Can you work these out from the drawing? Everything is in mm from the part's minimum corner. A direction names the side the tool comes from. Give positions to 0.01 mm unless a question says otherwise; leave off trailing zeros. Loops run counter-clockwise (first coordinate to the right, second up) from the corner with the lowest first, then second, coordinate; pieces in that order, holes last.
Q1. For the marked faces 4, 5, 6, 7 and 8, which set-ups out of +Z, -Z, +X, -X, +Y, -Y let a thin tool reach every point of the face, with its end or its side?
Q2. Will these pins go through, and if not, where does the flat tip stop? P1, Ø23.5, axis at x = 88, z = 17, coming from the -Y side (1 decimal); P2, Ø3, axis at y = 24.5, z = 14, coming from the -X side (1 decimal); P3, Ø8, axis at x = 99.5, z = 9.5, coming from the +Y side (1 decimal).
Q3. I need wall thicknesses on line 1 (Y direction, x = 115, z = 34) (1 decimal); line 2 (Z direction, x = 47, y = 15); line 3 (Y direction, x = 21.15, z = 6.5) (1 decimal). Which ranges of each line are inside material? Lowest first, please.
Q4. We'd pull the mould along Y, two halves only. Please class the marked faces 1, 2 and 3: +Y half, -Y half, draft (parallel to the pull), parting line (faces both ways), or undercut.
Q5. If we section it at D-D (z = 36): Please give me the cut outline in (x, y) (1 decimal), plus the area to 3 significant figures.
Q6. If we section it at C-C (y = 17.5): Please give me the cut outline in (x, z) (1 decimal).
Q7. If we section it at B-B (x = 21.15): Please give me the cut outline in (y, z) (1 decimal).
Q8. If we section it at A-A (y = 25.5): Please give me the cut outline in (x, z) (1 decimal).
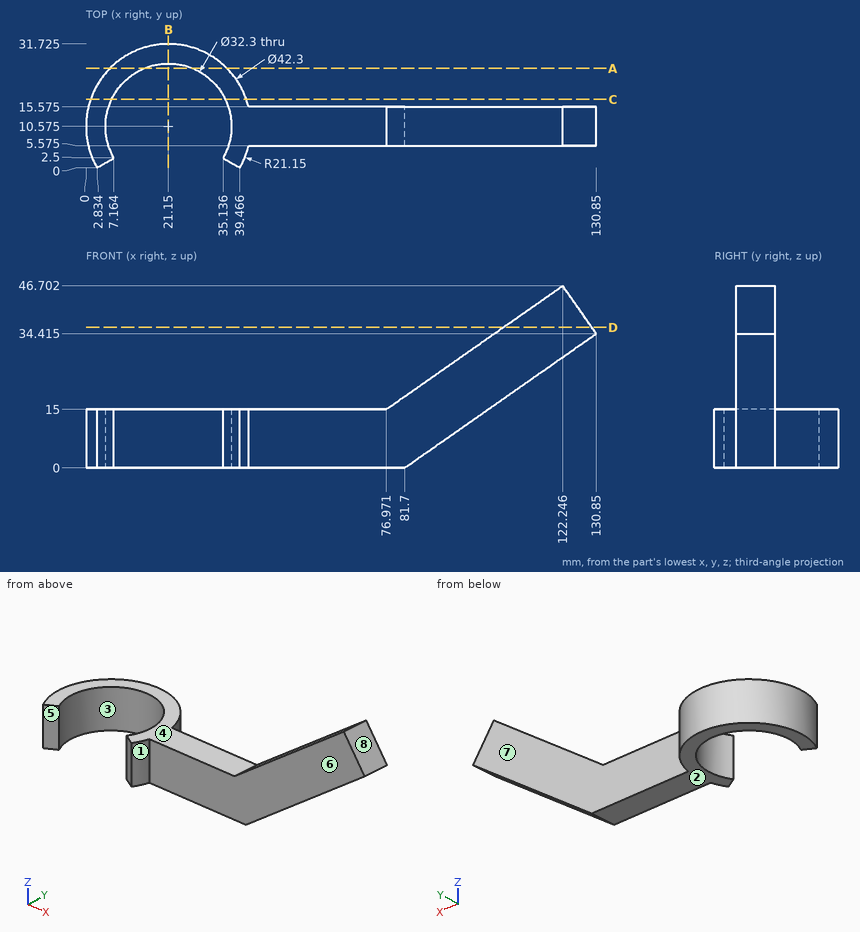
Check sheet entries:
1. face 4: +Z, -X, +Y, -Y
1. face 5: +Z, -Z, -Y
1. face 6: +Z, -Z, +X, -Y
1. face 7: +Z, -Z, +X, +Y
1. face 8: +Z, +X, +Y, -Y
2. P1: stops at y = 5.6
2. P2: stops at x = 4
2. P3: stops at y = 15.6
3. line 1: y = 5.6 to 15.6
3. line 2: z = 0 to 15
3. line 3: y = 26.7 to 31.7
4. face 1: -Y half
4. face 2: draft
4. face 3: undercut
5. outline: (107, 5.6) - (129.7, 5.6) - (129.7, 15.6) - (107, 15.6) - close
5. area: 228 mm2
6. outline: (1.2, 0) - (6.6, 0) - (6.6, 15) - (1.2, 15) - close; (35.7, 0) - (41.1, 0) - (41.1, 15) - (35.7, 15) - close
7. outline: (26.7, 0) - (31.7, 0) - (31.7, 15) - (26.7, 15) - close
8. outline: (6.2, 0) - (15, 0) - (15, 15) - (6.2, 15) - close; (27.3, 0) - (36.1, 0) - (36.1, 15) - (27.3, 15) - close
